Work out the finished part from the listing and answer in its coordinate system (mm). Face numbers are marked on the shaded views. A direction names the side the tool comes from. Coordinates: 2 decimals unless noted, no trailing zeros. Order: outer loops, then holes, each group sorted by start corner. A loop starts at its lowest first (then second) coordinate and runs counter-clockwise, first axis right, second up. Notation, with made-up numbers: M 7,4.5 L 53,4.5 A22 ccw 53,18.5 Z; hole C 1,46.5 d2. An arc over 180 degrees is marked long. Use a Markdown table: item, result.
from build123d import *

# Parameters (mm, degrees)
EXTRUDE_1_DEPTH     = 4
SKETCH_2_R          = 1.35
CUT_EXTRUDE_1_DEPTH = 4
CUT_EXTRUDE_2_DEPTH = 2
SKETCH_4_W          = 46
SKETCH_4_H          = 10
CUT_EXTRUDE_3_DEPTH = 2
SKETCH_6_W          = 10
SKETCH_6_H          = 25
CUT_EXTRUDE_4_DEPTH = 2
SKETCH_7_R          = 2
CUT_EXTRUDE_5_DEPTH = 2


with BuildPart() as part:
    # 草图1 → 凸台-拉伸1 (new body)
    with BuildSketch(Plane(origin=(0, 0, 0), x_dir=(1, 0, 0), z_dir=(0, 1, 0))):
        with BuildLine():
            Line((2.5, 0), (38.5, 0))
            ThreePointArc((38.5, 0), (40.267766953, 0.732233047), (41, 2.5))
            Line((41, 2.5), (41, 38.5))
            ThreePointArc((41, 38.5), (40.267766953, 40.267766953), (38.5, 41))
            Line((38.5, 41), (2.5, 41))
            ThreePointArc((2.5, 41), (0.732233047, 40.267766953), (0, 38.5))
            Line((0, 38.5), (0, 2.5))
            ThreePointArc((0, 2.5), (0.732233047, 0.732233047), (2.5, 0))
        make_face()
    extrude(amount=-EXTRUDE_1_DEPTH)

    # 草图2 → 切除-拉伸1 (cut)
    with BuildSketch(Plane.XZ.offset(4)):
        with Locations(Location((2.5, -2.5, 0), (0, 0, 270))):
            Circle(SKETCH_2_R)
        with Locations(Location((38.5, -2.5, 0), (0, 0, 90))):
            Circle(SKETCH_2_R)
        with Locations(Location((2.5, -38.5, 0), (0, 0, 90))):
            Circle(SKETCH_2_R)
        with Locations(Location((38.5, -38.5, 0), (0, 0, 270))):
            Circle(SKETCH_2_R)
    extrude(amount=-CUT_EXTRUDE_1_DEPTH, mode=Mode.SUBTRACT)

    # 草图3 → 切除-拉伸2 (cut)
    with BuildSketch(Plane.XZ.offset(4)):
        with BuildLine():
            Line((0, -10), (0, -13))
            ThreePointArc((0, -13), (0.878679656, -10.878679656), (3, -10))
            Line((3, -10), (7, -10))
            ThreePointArc((7, -10), (9.121320344, -9.121320344), (10, -7))
            Line((10, -7), (10, -3))
            ThreePointArc((10, -3), (10.878679656, -0.878679656), (13, 0))
            Line((13, 0), (10, 0))
            Line((10, 0), (0, 0))
            Line((0, 0), (0, -10))
        make_face()
        with BuildLine():
            Line((41, 0), (41, -10))
            Line((41, -10), (41, -13))
            ThreePointArc((41, -13), (40.121320344, -10.878679656), (38, -10))
            Line((38, -10), (34, -10))
            ThreePointArc((34, -10), (31.878679656, -9.121320344), (31, -7))
            Line((31, -7), (31, -3))
            ThreePointArc((31, -3), (30.121320344, -0.878679656), (28, 0))
            Line((28, 0), (31, 0))
            Line((31, 0), (41, 0))
        make_face()
        with BuildLine():
            Line((41, -41), (31, -41))
            Line((31, -41), (28, -41))
            ThreePointArc((28, -41), (30.121320344, -40.121320344), (31, -38))
            Line((31, -38), (31, -34))
            ThreePointArc((31, -34), (31.878679656, -31.878679656), (34, -31))
            Line((34, -31), (38, -31))
            ThreePointArc((38, -31), (40.121320344, -30.121320344), (41, -28))
            Line((41, -28), (41, -31))
            Line((41, -31), (41, -41))
        make_face()
        with BuildLine():
            Line((0, -41), (0, -31))
            Line((0, -31), (0, -28))
            ThreePointArc((0, -28), (0.878679656, -30.121320344), (3, -31))
            Line((3, -31), (7, -31))
            ThreePointArc((7, -31), (9.121320344, -31.878679656), (10, -34))
            Line((10, -34), (10, -38))
            ThreePointArc((10, -38), (10.878679656, -40.121320344), (13, -41))
            Line((13, -41), (10, -41))
            Line((10, -41), (0, -41))
        make_face()
    extrude(amount=-CUT_EXTRUDE_2_DEPTH, mode=Mode.SUBTRACT)

    # 草图4 → 切除-拉伸3 (cut)
    with BuildSketch(Plane(origin=(0, 0, 0), x_dir=(1, 0, 0), z_dir=(0, 1, 0))):
        with Locations((20.5, 20.5)):
            Rectangle(SKETCH_4_W, SKETCH_4_H)
    extrude(amount=-CUT_EXTRUDE_3_DEPTH, mode=Mode.SUBTRACT)

    # 草图6 → 切除-拉伸4 (cut)
    with BuildSketch(Plane(origin=(0, 0, 0), x_dir=(1, 0, 0), z_dir=(0, 1, 0))):
        with Locations((20.5, 38)):
            Rectangle(SKETCH_6_W, SKETCH_6_H)
        with Locations((20.5, 3)):
            Rectangle(SKETCH_6_W, SKETCH_6_H)
    extrude(amount=-CUT_EXTRUDE_4_DEPTH, mode=Mode.SUBTRACT)

    # 草图7 → 切除-拉伸5 (cut)
    with BuildSketch(Plane(origin=(0, 0, 0), x_dir=(1, 0, 0), z_dir=(0, 1, 0))):
        with Locations((15, 37.7)):
            Circle(SKETCH_7_R)
        with Locations((26, 3.3)):
            Circle(SKETCH_7_R)
        with Locations((26, 37.7)):
            Circle(SKETCH_7_R)
        with Locations((15, 3.3)):
            Circle(SKETCH_7_R)
    extrude(amount=-CUT_EXTRUDE_5_DEPTH, mode=Mode.SUBTRACT)


solid = part.part
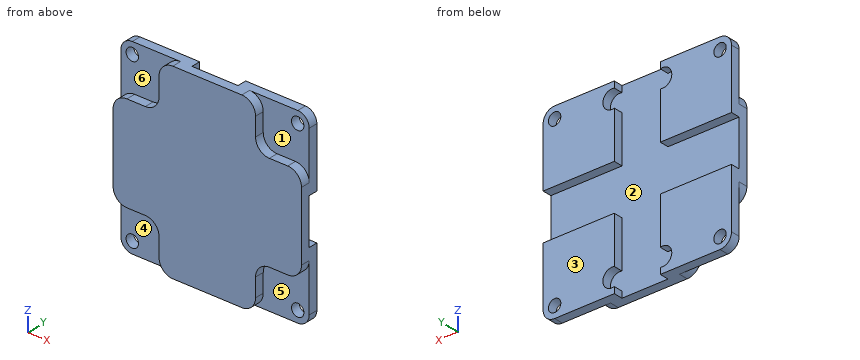
1. Flat-ended cylindrical pins translate along their axes: P1, Ø14.5, axis at x = 9, z = -6.5, coming from the -Y side; P2, Ø1.6, axis at y = -3, z = -6, coming from the +X side; P3, Ø1.5, axis at y = -1, z = -0.5, coming from the +X side; P4, Ø1, axis at x = 21, z = -18.5, coming from the +Y side. Find the tip coordinate at first contact, or state that the pin passes through.
Answers below:
| item | result |
|---|---|
| P1 | y = -4 |
| P2 | x = 31 |
| P3 | x = 40.67 |
| P4 | y = -2 |
2. Section C-C on y = -2.6 is taken. Determine the outline of the cut face in (x, z), then the cut area to 3 significant figures.
Answers below:
| item | result |
|---|---|
| outline | M 0,-28 A3 ccw 3,-31 L 7,-31 A3 cw 10,-34 L 10,-38 A3 ccw 13,-41 L 28,-41 A3 ccw 31,-38 L 31,-34 A3 cw 34,-31 L 38,-31 A3 ccw 41,-28 L 41,-13 A3 ccw 38,-10 L 34,-10 A3 cw 31,-7 L 31,-3 A3 ccw 28,0 L 13,0 A3 ccw 10,-3 L 10,-7 A3 cw 7,-10 L 3,-10 A3 ccw 0,-13 Z |
| area | 1,270 mm² |
3. Section B-B on z = -13.5 is taken. Determine the outline of the cut face in (x, y).
Answers below:
| item | result |
|---|---|
| outline | M 0,-4 L 41,-4 L 41,0 L 25.5,0 L 25.5,-2 L 15.5,-2 L 15.5,0 L 0,0 Z |
4. Section D-D on z = -2 is taken. Determine the outline of the cut face in (x, y), then the cut area to 3 significant figures.
Answers below:
| item | result |
|---|---|
| outline | M 0.05,-2 L 1.25,-2 L 1.25,0 L 0.05,0 Z; M 3.75,-2 L 10.17,-2 L 10.17,-4 L 30.83,-4 L 30.83,-2 L 37.25,-2 L 37.25,0 L 27.52,0 L 27.52,-2 L 13.48,-2 L 13.48,0 L 3.75,0 Z; M 39.75,-2 L 40.95,-2 L 40.95,0 L 39.75,0 Z |
| area | 85.0 mm² |
5. For a pull along X with two mould halves and no side action, classify the marked faces 1 and 2 as +X half, -X half, draft (parallel to the pull), parting line (faces both ways), or undercut.
Answers below:
| item | result |
|---|---|
| face 1 | draft |
| face 2 | undercut |
6. Find the intervals of material crossed by probe 1 along Z at (x, y) = (26, -0.8); probe 2 along X at (y, z) = (-0.3, -10.5); probe 3 along X at (y, z) = (-1.5, -38.5), in increasing order.
Answers below:
| item | result |
|---|---|
| probe 1 | -41 to -39.7, -35.7 to -25.5, -15.5 to -5.3, -1.3 to 0 |
| probe 2 | 0 to 15.5, 25.5 to 41 |
| probe 3 | 0 to 1.15, 3.85 to 13.17, 27.83 to 37.15, 39.85 to 41 |
7. For the marked faces 3, 4, 5 and 6, determine the directions among +Z, -Z, +X, -X, +Y, -Y from which every point of the face is accessible in a straight line to the end or side of a thin tool.
Answers below:
| item | result |
|---|---|
| face 3 | +Z, -Z, +X, -X, +Y |
| face 4 | -Z, -X, -Y |
| face 5 | -Z, +X, -Y |
| face 6 | +Z, -X, -Y |
8. Section A-A on x = 15 is taken. Determine the outline of the cut face in (y, z), then the cut area to 3 significant figures.
Answers below:
| item | result |
|---|---|
| outline | M -4,-41 L 0,-41 L 0,-39.7 L -2,-39.7 L -2,-35.7 L 0,-35.7 L 0,-25.5 L -2,-25.5 L -2,-15.5 L 0,-15.5 L 0,-5.3 L -2,-5.3 L -2,-1.3 L 0,-1.3 L 0,0 L -4,0 Z |
| area | 128 mm² |
